Read the model definition and answer for the solid it produces. Units are mm, in the model's axes. Face numbers are marked on the shaded views. A direction names the side the tool comes from. Give positions to 0.01 mm unless a question says otherwise; leave off trailing zeros. Loops run counter-clockwise (first coordinate to the right, second up) from the corner with the lowest first, then second, coordinate; pieces in that order, holes last.
(1) Find section B-B, the plane y = 219.95. Write down the section's boundary in (x, z), then the cut area to 3 significant figures.
(2) Each of these flat-tipped pins is pushed along its axis until it touches: P1, Ø2, axis at y = 211.5, z = -0.5, coming from the +X side; P2, Ø5, axis at x = 4, z = -5.5, coming from the +Y side; P3, Ø8, axis at y = 214.5, z = 1, coming from the +X side; P4, Ø2.5, axis at x = -5.61, y = 214.34, coming from the +Z side. Where does it stop, or does it pass through?
(3) Which of the six approach directions +Z, -Z, +X, -X, +Y, -Y give full straight-line access (tool end or side, diameter ignored) to the marked faces 1 and 2?
(4) Find section C-C, the plane y = 214. Write down the section's boundary in (x, z), then the cut area to 3 significant figures.
(5) Find section D-D, the plane x = -5.5. Write down the section's boundary in (y, z).
(6) Determine the mould class of the marked faces 3, 4, 5 and 6 for opening direction X: pulls with the +X half, pulls with the -X half, needs draft (parallel to the pull), parting line crosses it, or undercut.
(7) Straight lines are drawn through the part: probe 1 along Y at (x, z) = (0.25, -4.5) (3 decimals); probe 2 along Z at (x, y) = (-4.25, 224.75); probe 3 along X at (y, z) = (220, -1.5). For each, find the intervals that lie inside material, in ascending order.
(8) Find section A-A, the plane x = 0.05. Write down the section's boundary in (y, z), then the cut area to 3 significant figures.
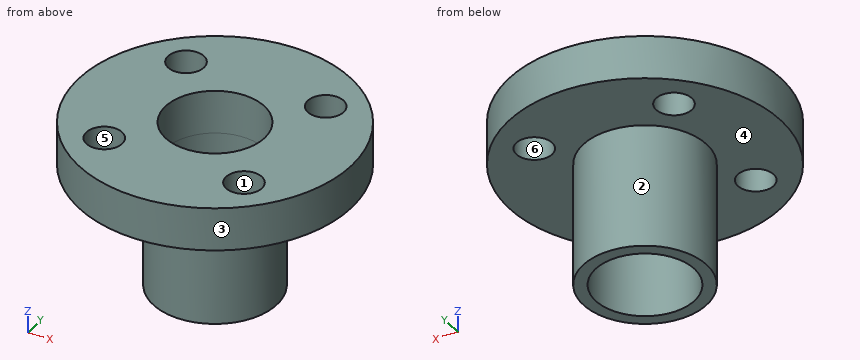
```python
from build123d import *

# Parameters (mm, degrees)
SKETCH1_R           = 11
SKETCH1_R_2         = 4
SKETCH1_R_3         = 1.45
BOSS_EXTRUDE1_DEPTH = 3.5
SKETCH2_R           = 5
SKETCH2_R_2         = 4
BOSS_EXTRUDE2_DEPTH = 10


with BuildPart() as part:
    # Sketch1 → Boss-Extrude1 (new body)
    with BuildSketch(Plane.XY):
        with Locations((0.049999962, 219.95)):
            Circle(SKETCH1_R)
        with Locations((0.049999962, 219.95)):
            Circle(SKETCH1_R_2, mode=Mode.SUBTRACT)
        with Locations((5.656854228, 214.293145824)):
            Circle(SKETCH1_R_3, mode=Mode.SUBTRACT)
        with Locations((-5.606854214, 214.343145734)):
            Circle(SKETCH1_R_3, mode=Mode.SUBTRACT)
        with Locations((-5.556854304, 225.606854176)):
            Circle(SKETCH1_R_3, mode=Mode.SUBTRACT)
        with Locations((5.706854138, 225.556854266)):
            Circle(SKETCH1_R_3, mode=Mode.SUBTRACT)
    extrude(amount=BOSS_EXTRUDE1_DEPTH)

    # Sketch2 → Boss-Extrude2 (add)
    with BuildSketch(Plane(origin=(0, 0, 0), x_dir=(-1, 0, 0), z_dir=(0, 0, -1))):
        with Locations((-0.049999962, 219.95)):
            Circle(SKETCH2_R)
        with Locations((-0.049999962, 219.95)):
            Circle(SKETCH2_R_2, mode=Mode.SUBTRACT)
    extrude(amount=BOSS_EXTRUDE2_DEPTH)


solid = part.part
```
Entries:
1. outline: (-10.95, 0) - (-4.95, 0) - (-4.95, -10) - (-3.95, -10) - (-3.95, 3.5) - (-10.95, 3.5) - close; (4.05, -10) - (5.05, -10) - (5.05, 0) - (11.05, 0) - (11.05, 3.5) - (4.05, 3.5) - close
1. area: 69.0 mm2
2. P1: stops at x = 8.02
2. P2: stops at y = 224.74
2. P3: stops at x = 10.95
2. P4: passes through
3. face 1: +Z, -Z
3. face 2: -Z
4. outline: (-9.2, 0) - (-7.02, 0) - (-7.02, 3.5) - (-9.2, 3.5) - close; (-4.2, 0) - (4.24, 0) - (4.24, 3.5) - (-4.2, 3.5) - close; (7.08, 0) - (9.3, 0) - (9.3, 3.5) - (7.08, 3.5) - close
4. area: 45.0 mm2
5. outline: (210.45, 0) - (212.9, 0) - (212.9, 3.5) - (210.45, 3.5) - close; (215.79, 0) - (224.16, 0) - (224.16, 3.5) - (215.79, 3.5) - close; (227.06, 0) - (229.45, 0) - (229.45, 3.5) - (227.06, 3.5) - close
6. face 3: parting line crosses it
6. face 4: needs draft
6. face 5: undercut
6. face 6: undercut
7. probe 1: y = 214.954 to 215.955, 223.945 to 224.946
7. probe 2: z = 0 to 3.5
7. probe 3: x = -4.95 to -3.95, 4.05 to 5.05
8. outline: (208.95, 0) - (214.95, 0) - (214.95, -10) - (215.95, -10) - (215.95, 3.5) - (208.95, 3.5) - close; (223.95, -10) - (224.95, -10) - (224.95, 0) - (230.95, 0) - (230.95, 3.5) - (223.95, 3.5) - close
8. area: 69.0 mm2
